Model file for the job. Use its own axes, mm. Round coordinates to 2 decimals unless told otherwise and drop trailing zeros. Loops run counter-clockwise (first coordinate to the right, second up) from the corner with the lowest first, then second, coordinate; pieces in that order, holes last. Notation, with made-up numbers: (75, 42) - (92, 42) arc R18 ccw to (92, 72) - close; hole circle Ø9 at (15, -18.75). An arc over 180 degrees is marked (long way). Use one line per item in the form item = value.
from build123d import *

# Parameters (mm, degrees)
BASE_FLANGE1_DEPTH = 1
SKETCH2_R          = 3
CUT_EXTRUDE1_DEPTH = 10
FILLET1_R          = 3


# Sheet-metal steps are written as plain solids
with BuildPart() as part:
    # Sketch1 → Base-Flange1 (new body)
    with BuildSketch(Plane.XY):
        Polygon((104, 853), (16, 853), (16, 107.151941455), (170, 18.24), (170, 123.634882233), (104, 161.74), align=None)
    extrude(amount=-BASE_FLANGE1_DEPTH)

    # Sketch2 → Cut-Extrude1 (cut)
    with BuildSketch(Plane(origin=(0, 0, -1), x_dir=(-1, 0, 0), z_dir=(0, 0, -1))):
        with Locations((-22, 824)):
            Circle(SKETCH2_R)
        with Locations((-98, 824)):
            Circle(SKETCH2_R)
        with Locations((-98, 656)):
            Circle(SKETCH2_R)
        with Locations((-98, 488)):
            Circle(SKETCH2_R)
        with Locations((-98, 320)):
            Circle(SKETCH2_R)
        with Locations((-22, 656)):
            Circle(SKETCH2_R)
        with Locations((-22, 488)):
            Circle(SKETCH2_R)
        with Locations((-22, 320)):
            Circle(SKETCH2_R)
        with Locations((-22, 152)):
            Circle(SKETCH2_R)
        with Locations((-98, 177)):
            Circle(SKETCH2_R)
        with Locations((-140, 134.564882233)):
            Circle(SKETCH2_R)
        with Locations((-130, 50.734882233)):
            Circle(SKETCH2_R)
        with Locations((-43.397459622, 100.734882233)):
            Circle(SKETCH2_R)
    extrude(amount=-CUT_EXTRUDE1_DEPTH, mode=Mode.SUBTRACT)

    # Fillet1
    fillet1_edges = [part.edges().sort_by_distance(p)[0] for p in [
        (104, 161.74, -0.5),
        (170, 123.634882233, -0.5),
        (170, 18.24, -0.5),
        (16, 107.151941455, -0.5),
        (16, 853, -0.5),
        (104, 853, -0.5),
    ]]
    fillet(fillet1_edges, radius=FILLET1_R)


solid = part.part
1. Wall check: probe 1 along X at (y, z) = (488, -0.55); probe 2 along Y at (x, z) = (22, -0.7); probe 3 along X at (y, z) = (177, -0.35). Give the ranges that are in metal, low to high.
Geometry check:
probe_1 = 16 to 19, 25 to 95, 101 to 104
probe_2 = 103.69 to 149, 155 to 317, 323 to 485, 491 to 653, 659 to 821, 827 to 853
probe_3 = 16 to 95, 101 to 104
2. Flat gauge pin, fed straight in: pin 1 (3.5 mm diameter, centred on x = 98, y = 488, fed in from -Z). Where does the tip first touch, or does it go through?
Geometry check:
pin_1 = through
3. Pull direction Z, two halves, no side cores. Call faces 1 (the flat face through (90.464, 64.16, -0.493)), 2 (the flat face through (58, 443, 0)), 3 (the flat face through (58, 443, -1)): +Z half, -Z half, draft (parallel to the pull), parting line (faces both ways), or undercut.
Geometry check:
face_1 = draft
face_2 = +Z half
face_3 = -Z half
4. Cut at C-C, the plane x = 155. Give the cut face in (y, z).
Geometry check:
outline = (26.9, -1) - (132.3, -1) - (132.3, 0) - (26.9, 0) - close
5. Cut at B-B, the plane y = 386.5. Give the cut face in (x, z).
Geometry check:
outline = (16, -1) - (104, -1) - (104, 0) - (16, 0) - close
6. Cut at A-A, the plane z = -0.2. Give the number of separate pieces and of enclosed holes in the cut face, plus the area to 3 significant figures.
Geometry check:
separate_pieces = 1
enclosed_holes = 13
area = 74,400 mm^2
